```python
from build123d import *

# Parameters (mm, degrees)
CROQUIS2_R            = 0.5
CROQUIS2_W            = 4
CROQUIS2_H            = 5
CORTAR_EXTRUIR1_DEPTH = 6


with BuildPart() as part:
    # Croquis1 → Revolución1 (revolve)
    with BuildSketch(Plane.XY):
        with BuildLine():
            ThreePointArc((9.25, 7.5), (8.517766953, 5.732233047), (6.75, 5))
            Line((6.75, 5), (0, 5))
            Line((0, 5), (0, 0))
            Line((0, 0), (9.25, 0))
            Line((9.25, 0), (9.25, 7.5))
        make_face()
    revolve(axis=Axis((0, 0, 0), (0, 1, 0)))

    # Croquis2 → Cortar-Extruir1 (cut, through all)
    with BuildSketch(Plane(origin=(0, 5, 0), x_dir=(1, 0, 0), z_dir=(0, 1, 0))):
        with Locations((0, 5.75)):
            Circle(CROQUIS2_R)
        with Locations((2.672158239, 5.091372148)):
            Circle(CROQUIS2_R)
        with Locations((4.732157229, 3.266372294)):
            Circle(CROQUIS2_R)
        with Locations((5.708076026, 0.693085911)):
            Circle(CROQUIS2_R)
        with Locations((5.376343395, -2.0389781)):
            Circle(CROQUIS2_R)
        with Locations((3.812955285, -4.303936802)):
            Circle(CROQUIS2_R)
        with Locations((1.37606507, -5.58291545)):
            Circle(CROQUIS2_R)
        with Locations((-1.37606507, -5.58291545)):
            Circle(CROQUIS2_R)
        with Locations((-3.812955285, -4.303936802)):
            Circle(CROQUIS2_R)
        with Locations((-5.376343395, -2.0389781)):
            Circle(CROQUIS2_R)
        with Locations((-5.708076026, 0.693085911)):
            Circle(CROQUIS2_R)
        with Locations((-4.732157229, 3.266372294)):
            Circle(CROQUIS2_R)
        with Locations((-2.672158239, 5.091372148)):
            Circle(CROQUIS2_R)
        Rectangle(CROQUIS2_W, CROQUIS2_H)
    extrude(amount=-CORTAR_EXTRUIR1_DEPTH, mode=Mode.SUBTRACT)


solid = part.part
```
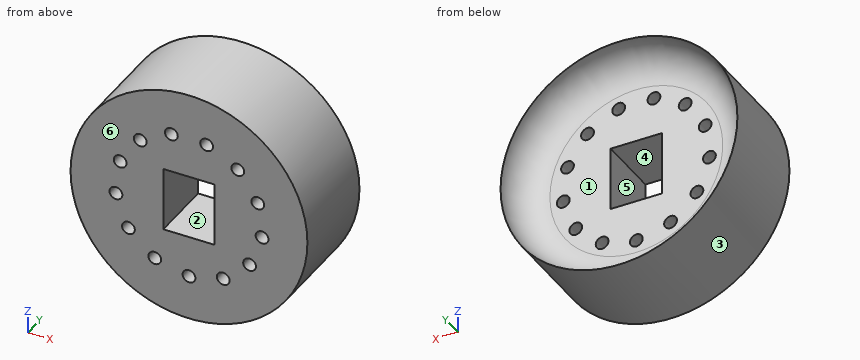
Verification items for the finished model (mm, model axes). Face numbers are marked on the shaded views. A direction names the side the tool comes from. Give positions to 0.01 mm unless a question says otherwise; leave off trailing zeros. Write each loop counter-clockwise with the first axis right and the second up, starting at its lowest first coordinate (ties: lowest second). Pieces come first, ordered by that corner, then holes. Notation, with made-up numbers: M 87,41.25 L 132,41.25 A7 ccw 132,46.25 Z; hole C -38.75,-26.75 d7. An arc over 180 degrees is marked long. One line per question, with ' | ' between items.
1) Section check B-B on y = 1.5. State how many separate pieces and enclosed holes the cut face has, plus the area to 3 significant figures.
Result:
separate pieces: 1 | enclosed holes: 14 | area: 239 mm2
2) Thickness scan on line 1 along Z through (x, y) = (0, 1.7); line 2 along X through (y, z) = (2.5, 5.5); line 3 along X through (y, z) = (3.75, 5.25). Record the ranges inside material, lowest first. Write a range as [from, to].
Result:
line 1: z = [-9.25, -6.25], [-5.25, -2.5], [2.5, 9.25] | line 2: x = [-7.44, -1.87], [-0.88, 0.88], [1.87, 7.44] | line 3: x = [-7.62, -1.75], [-1, 1], [1.75, 7.62]
3) Section check D-D on y = 6.5. Enter the section's corners in (x, z).
Result:
outline: C 0,0 d18.5; hole C 0,0 d18.08
4) Gauge pin test, flat ends, axial feed: pin 1 Ø3 at (y, z) = (6.5, 3) entering from +X; pin 2 Ø2 at (x, y) = (-3.5, 2) entering from +Z; pin 3 Ø1.5 at (y, z) = (2, 3) entering from +X. Record the tip position at first contact, or that the pin passes through.
Result:
pin 1: stops at x = 9.13 | pin 2: stops at z = 8.91 | pin 3: stops at x = 8.97
5) Section check A-A on x = 0. Enter the section's corners in (y, z), plus the area to 3 significant figures.
Result:
outline: M 0,-9.25 L 7.5,-9.25 A2.5 cw 5,-6.75 L 5,-6.25 L 0,-6.25 Z; M 0,-5.25 L 5,-5.25 L 5,-2.5 L 0,-2.5 Z; M 0,2.5 L 5,2.5 L 5,6.75 A2.5 cw 7.5,9.25 L 0,9.25 Z | area: 65.2 mm2
6) Set-up check for the marked faces 1 and 2: record each of +Z, -Z, +X, -X, +Y, -Y from which the full face is reachable in a straight line by a thin tool's end or side.
Result:
face 1: +Y | face 2: +Y, -Y
7) Mould release check, pull along Z, two halves, no side actions. Record for the marked faces 3, 4, 5 and 6: released by +Z, released by -Z, zero draft, split by the parting line, or undercut.
Result:
face 3: split by the parting line | face 4: undercut | face 5: undercut | face 6: zero draft
8) Section check C-C on y = 5.5. Enter the section's corners in (x, z), plus the area to 3 significant figures.
Result:
outline: C 0,0 d18.5; hole C 0,0 d16.5 | area: 55.0 mm2
